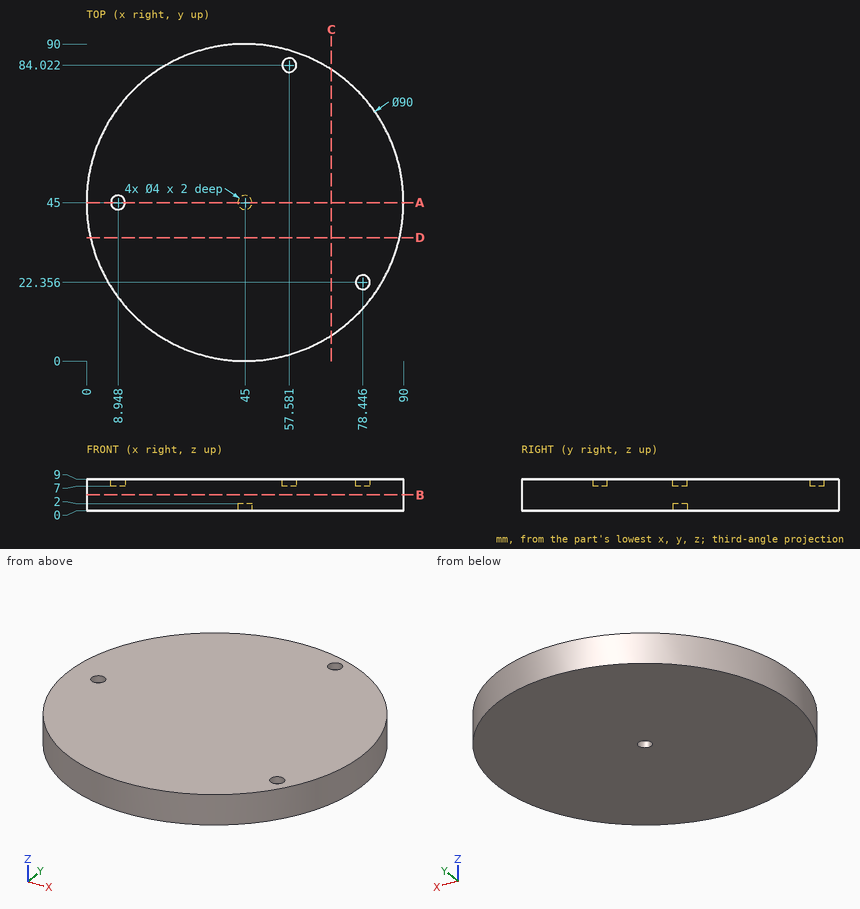
The drawing under review shows one solid part. Ordinate dimensions are in mm from its lowest x, y, z. Give positions to 0.01 mm unless a question says otherwise; leave off trailing zeros. Order: outer loops, then holes, each group sorted by start corner. A loop starts at its lowest first (then second) coordinate and runs counter-clockwise, first axis right, second up. Notation, with made-up numbers: (19.25, 41) - (48.25, 41) arc R17 ccw to (48.25, 67) - close; hole circle Ø3 at (33.5, 16.25). An arc over 180 degrees is marked (long way). Answer as a JSON object with one key per item and string values. Group by question number.
Item 1: Wall thickness on line 1 along Y through (x, z) = (45, 1); line 2 along Y through (x, z) = (44.5, 6.75); line 3 along X through (y, z) = (17, 6.25): over which ranges is each line inside the solid? List them lowest first.
Item 2: Take a section at A-A on y = 45. Give the boundary of the cut face in (x, z).
Item 3: Take a section at C-C on x = 69.5. Give the boundary of the cut face in (y, z) (1 decimal).
Item 4: Take a section at D-D on y = 35. Give the boundary of the cut face in (x, z) (1 decimal), and give its area (3 significant figures).
Item 5: Clearance check with flat-ended pins moving along their axes: pin 1 Ø3 at (x, y) = (58, 84) entering from +Z; pin 2 Ø5 at (y, z) = (63.5, 2) entering from +X. State where each tip first meets the part, or that it passes through.
Item 6: Take a section at B-B on z = 4.5. Give the boundary of the cut face in (x, y), and give its area (3 significant figures).
Reported:
{
 "1": {"line 1": "0 to 43, 47 to 90", "line 2": "0 to 90", "line 3": "9.77 to 80.23"},
 "2": {"outline": "(0, 0) - (43, 0) - (43, 2) - (47, 2) - (47, 0) - (90, 0) - (90, 9) - (10.95, 9) - (10.95, 7) - (6.95, 7) - (6.95, 9) - (0, 9) - close"},
 "3": {"outline": "(7.3, 0) - (82.7, 0) - (82.7, 9) - (7.3, 9) - close"},
 "4": {"outline": "(1.1, 0) - (88.9, 0) - (88.9, 9) - (1.1, 9) - close", "area": "790 mm^2"},
 "5": {"pin 1": "z = 7", "pin 2": "x = 87.06"},
 "6": {"outline": "circle Ø90 at (45, 45)", "area": "6,360 mm^2"}
}
